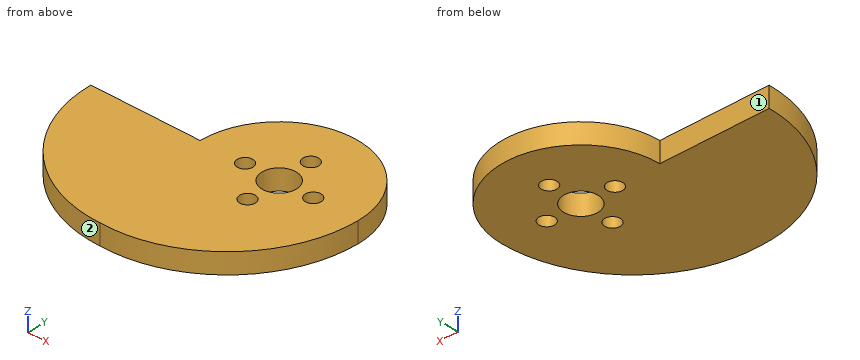
from build123d import *

# Parameters (mm, degrees)
SKETCH1_R             = 4
BOSS_EXTRUDE1_DEPTH   = 4.7625
F_6_CLEARANCE_HOLE1_D = 3.6576


with BuildPart() as part:
    # Sketch1 → Boss-Extrude1 (new body)
    with BuildSketch(Plane.XY):
        with BuildLine():
            Line((-44.196, 0), (-18.542, 0))
            ThreePointArc((-18.542, 0), (0, 18.542), (18.542, 0))
            ThreePointArc((18.542, 0), (9.088190436, -22.185776818), (-13.462, -30.734))
            ThreePointArc((-13.462, -30.734), (-35.194219813, -21.732219813), (-44.196, 0))
        make_face()
        Circle(SKETCH1_R, mode=Mode.SUBTRACT)
    extrude(amount=BOSS_EXTRUDE1_DEPTH)

    # #6 Clearance Hole1 (through all)
    with Locations(Plane.XY.offset(4.7625)):
        with Locations((0, 8), (8, 0), (0, -8), (-8, 0)):
            Hole(F_6_CLEARANCE_HOLE1_D / 2)


solid = part.part
Geometry check sheet. Reference: the model listing, model coordinates, mm. Face numbers are marked on the shaded views. A direction names the side the tool comes from. Give positions to 0.01 mm unless a question says otherwise; leave off trailing zeros. Order: outer loops, then holes, each group sorted by start corner. A loop starts at its lowest first (then second) coordinate and runs counter-clockwise, first axis right, second up.
1) Cross-section at B-B (x = -8). Record the boundary of the cut face in (y, z), then the cut area to 3 significant figures.
Results are:
outline: (-30.47, 0) - (-1.83, 0) - (-1.83, 4.76) - (-30.47, 4.76) - close; (1.83, 0) - (16.73, 0) - (16.73, 4.76) - (1.83, 4.76) - close
area: 207 mm2
2) Gauge pin test, flat ends, axial feed: pin 1 (2 mm diameter, centred on x = -22, z = 1.5, fed in from -Y); pin 2 (9 mm diameter, centred on x = 0, y = 0, fed in from -Z); pin 3 (1 mm diameter, centred on y = 5, z = 2.5, fed in from +X). Record the tip position at first contact, or that the pin passes through.
Results are:
pin 1: stops at y = -29.8
pin 2: stops at z = 0
pin 3: stops at x = 17.99
3) Tool access check on the marked faces 1 and 2. Record the directions out of +Z, -Z, +X, -X, +Y, -Y that give a thin tool (end or side, any length) a straight path to the whole face; none if there is none.
Results are:
face 1: +Z, -Z, -X, +Y
face 2: +Z, -Z, -X, -Y
4) Cross-section at D-D (x = 0). Record the boundary of the cut face in (y, z).
Results are:
outline: (-28.23, 0) - (-9.83, 0) - (-9.83, 4.76) - (-28.23, 4.76) - close; (-6.17, 0) - (-4, 0) - (-4, 4.76) - (-6.17, 4.76) - close; (4, 0) - (6.17, 0) - (6.17, 4.76) - (4, 4.76) - close; (9.83, 0) - (18.54, 0) - (18.54, 4.76) - (9.83, 4.76) - close
5) Cross-section at C-C (y = -8). Record the boundary of the cut face in (x, z), then the cut area to 3 significant figures.
Results are:
outline: (-43.14, 0) - (-1.83, 0) - (-1.83, 4.76) - (-43.14, 4.76) - close; (1.83, 0) - (17.48, 0) - (17.48, 4.76) - (1.83, 4.76) - close
area: 271 mm2
6) Material ranges on probe 1 along Y at (x, z) = (0, 1.6); probe 2 along X at (y, z) = (1, 2.6); probe 3 along X at (y, z) = (7, 2.85), recorded low to high.
Results are:
probe 1: y = -28.23 to -9.83, -6.17 to -4, 4 to 6.17, 9.83 to 18.54
probe 2: x = -18.52 to -9.53, -6.47 to -3.87, 3.87 to 6.47, 9.53 to 18.52
probe 3: x = -17.17 to -1.53, 1.53 to 17.17
7) Cross-section at A-A (z = 3.75). Record the boundary of the cut face in (x, y).
Results are:
outline: (-44.2, 0) arc R30.73 ccw to (-13.46, -30.73) arc R30.76 ccw to (18.54, 0) arc R18.54 ccw to (-18.54, 0) - close; hole circle Ø3.66 at (-8, 0); hole circle Ø8 at (0, 0); hole circle Ø3.66 at (0, -8); hole circle Ø3.66 at (0, 8); hole circle Ø3.66 at (8, 0)
